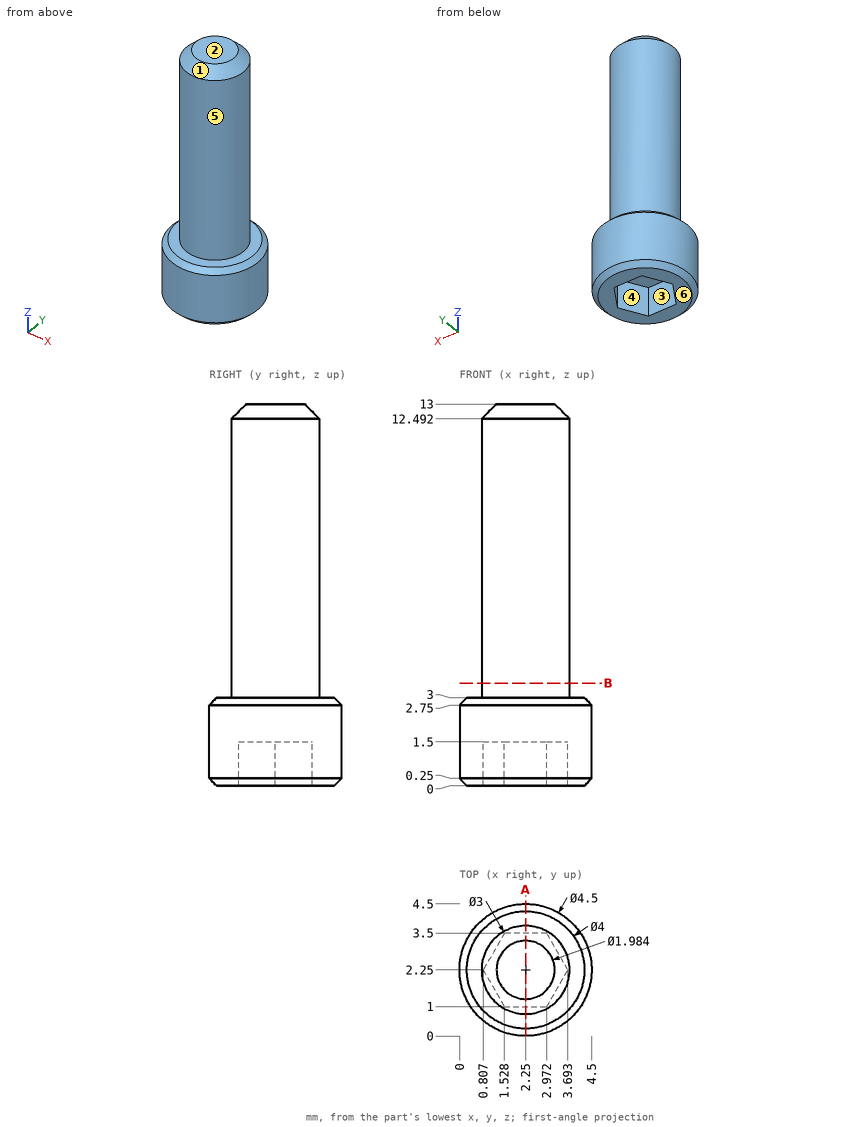
For this review, use the dimensioned drawing (mm, ordinates from the lowest corner) and the shaded views. A direction names the side the tool comes from. Coordinates: 2 decimals unless noted, no trailing zeros. Order: outer loops, then holes, each group sorted by start corner. A loop starts at its lowest first (then second) coordinate and runs counter-clockwise, first axis right, second up. Notation, with made-up numbers: M 59,-36 L 108,-36 A23 ccw 108,-20 Z; hole C 58.5,60 d5. An arc over 180 degrees is marked long. Answer as a JSON object with one key per item and string values. Group by question number.
1) Mouldability with a two-part tool opening along Y and no side actions: class the marked faces 1, 2, 3 and 4 as pulls with the +Y half, pulls with the -Y half, needs draft (parallel to the pull), parting line crosses it, or undercut.
2) Tool access review of the marked faces 5 and 6: name each direction out of +Z, -Z, +X, -X, +Y, -Y from which nothing blocks a thin tool from reaching the whole face with its end or side.
3) Wall thickness on L1, parallel to X at y = 2.65, z = 12 (1 decimal); L2, parallel to Z at x = 2.95, y = 3.65; L3, parallel to Z at x = 2.1, y = 1.9: over which ranges is each line inside the solid? List them lowest first.
4) Add section B-B, the plane z = 3.5. Write out the cut boundary in (x, y).
5) Add section A-A, the plane x = 2.25. Write out the cut boundary in (y, z).
Computed values:
{
 "1": {"face 1": "parting line crosses it", "face 2": "needs draft", "face 3": "undercut", "face 4": "undercut"},
 "2": {"face 5": "+Z", "face 6": "-Z, +X, -X, +Y, -Y"},
 "3": {"L1": "x = 0.8 to 3.7", "L2": "z = 0 to 3", "L3": "z = 1.5 to 13"},
 "4": {"outline": "C 2.25,2.25 d3"},
 "5": {"outline": "M 0,0.25 L 0.25,0 L 1,0 L 1,1.5 L 3.5,1.5 L 3.5,0 L 4.25,0 L 4.5,0.25 L 4.5,2.75 L 4.25,3 L 3.75,3 L 3.75,12.49 L 3.24,13 L 1.26,13 L 0.75,12.49 L 0.75,3 L 0.25,3 L 0,2.75 Z"}
}
